The listing builds one solid part. Answer for the finished solid, in the listing's coordinates (mm). Coordinates: 2 decimals unless noted, no trailing zeros. Loops run counter-clockwise (first coordinate to the right, second up) from the corner with the lowest first, then second, coordinate; pieces in that order, holes last. Notation, with made-up numbers: M 54,46.5 L 75,46.5 A12 cw 75,65.5 Z; hole C 45,68.25 d9. An arc over 180 degrees is marked long. Return JSON: item names as keys, results as strings. Group by question number.
1. Section C-C (z = 97.5) is taken. Write down the section's boundary in (x, y).
2. Section A-A (y = 0) is taken. Write down the section's boundary in (x, z).
3. Straight lines are drawn through the part: L1, parallel to Z at x = 5, y = -2; L2, parallel to Y at x = -1, z = -99. For each, find the intervals that lie inside material, in ascending order. Write a range as from..to.
4. Section B-B (x = 6.5) is taken. Write down the section's boundary in (y, z).
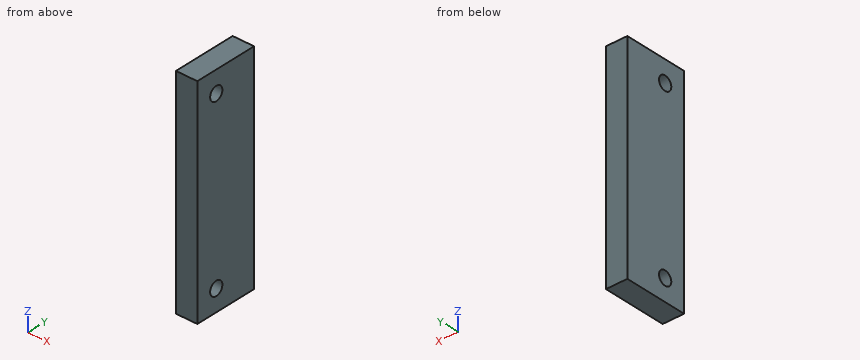
```python
from build123d import *

# Parameters (mm, degrees)
SKETCH1_W      = 257.175
SKETCH1_H      = 76.2
SKETCH1_R      = 8.227896341
EXTRUDE1_DEPTH = 12.7


with BuildPart() as part:
    # Sketch1 → Extrude1 (new, symmetric)
    with BuildSketch(Plane(origin=(0, 0, 0), x_dir=(0, 0, -1), z_dir=(1, 0, 0))):
        with Locations((0, 12.7)):
            Rectangle(SKETCH1_W, SKETCH1_H)
        with Locations((-103.1875, 0)):
            Circle(SKETCH1_R, mode=Mode.SUBTRACT)
        with Locations((103.1875, 0)):
            Circle(SKETCH1_R, mode=Mode.SUBTRACT)
    extrude(amount=EXTRUDE1_DEPTH, both=True)


solid = part.part
```
Worked out:
{
 "1": {"outline": "M -12.7,-25.4 L 12.7,-25.4 L 12.7,-5.95 L -12.7,-5.95 Z; M -12.7,5.95 L 12.7,5.95 L 12.7,50.8 L -12.7,50.8 Z"},
 "2": {"outline": "M -12.7,-128.59 L 12.7,-128.59 L 12.7,-111.42 L -12.7,-111.42 Z; M -12.7,-94.96 L 12.7,-94.96 L 12.7,94.96 L -12.7,94.96 Z; M -12.7,111.42 L 12.7,111.42 L 12.7,128.59 L -12.7,128.59 Z"},
 "3": {"L1": "-128.59..-111.17, -95.21..95.21, 111.17..128.59", "L2": "-25.4..-7.08, 7.08..50.8"},
 "4": {"outline": "M -25.4,-128.59 L 50.8,-128.59 L 50.8,128.59 L -25.4,128.59 Z; hole C 0,-103.19 d16.46; hole C 0,103.19 d16.46"}
}
